from build123d import *

# Parameters (mm, degrees)
CROQUIS1_R              = 2
CROQUIS1_R_2            = 6
CROQUIS1_R_3            = 1
SALIENTE_EXTRUIR1_DEPTH = 6


with BuildPart() as part:
    # Croquis1 → Saliente-Extruir1 (new body)
    with BuildSketch(Plane.XY):
        with BuildLine():
            Line((-26.32, 5.852999231), (-2.53, 11.218248526))
            ThreePointArc((-2.53, 11.218248526), (0, 11.5), (2.53, 11.218248526))
            Line((2.53, 11.218248526), (26.32, 5.852999231))
            ThreePointArc((26.32, 5.852999231), (31, 0), (26.32, -5.852999231))
            Line((26.32, -5.852999231), (2.53, -11.218248526))
            ThreePointArc((2.53, -11.218248526), (0, -11.5), (-2.53, -11.218248526))
            Line((-2.53, -11.218248526), (-26.32, -5.852999231))
            ThreePointArc((-26.32, -5.852999231), (-31, 0), (-26.32, 5.852999231))
        make_face()
        with Locations((-25, 0)):
            Circle(CROQUIS1_R, mode=Mode.SUBTRACT)
        Circle(CROQUIS1_R_2, mode=Mode.SUBTRACT)
        with Locations((-16, 0)):
            Circle(CROQUIS1_R_3, mode=Mode.SUBTRACT)
        with Locations(Location((16, 0, 0), (0, 0, 180))):
            Circle(CROQUIS1_R_3, mode=Mode.SUBTRACT)
    extrude(amount=SALIENTE_EXTRUIR1_DEPTH)


solid = part.part
Part model, mm, in its own coordinate system. Give positions to 0.01 mm unless a question says otherwise; leave off trailing zeros. Loops run counter-clockwise (first coordinate to the right, second up) from the corner with the lowest first, then second, coordinate; pieces in that order, holes last. Notation, with made-up numbers: (51, -9) -> (77, -9) arc R26 ccw to (77, 28) -> close; hole circle Ø9 at (87, -7.5). An arc over 180 degrees is marked (long way). Write each question's results on one line, items separated by ' | '. Start each with the question number.
Q1. Pin check, flat tips, straight feed: P1, Ø6, axis at x = 23.5, y = 1.5, coming from the -Z side; P2, Ø3, axis at y = -3, z = 1, coming from the -X side; P3, Ø11, axis at x = 0, y = 0, coming from the -Z side. Stop position of each tip, or through.
Q2. Wall check: L1, parallel to Y at x = 0, z = 2.1; L2, parallel to Y at x = 5.5, z = 1.65; L3, parallel to X at y = -4, z = 2.05. Give the ranges that are in metal, low to high.
Q3. Band-saw the part on B-B on x = 0. List the corners of the cut face in (y, z), plus the area to 3 significant figures.
Q4. Band-saw the part on C-C on y = 0. List the corners of the cut face in (x, z).
Q5. Band-saw the part on D-D on y = -4. List the corners of the cut face in (x, z).
Q6. Pull direction Y, two halves, no side cores. Call faces 1 (the face through (14.258, 8.573, 2.958)), 2 (the face through (0, -11.5, 3)), 3 (the face through (-15, 0, 3)): +Y half, -Y half, draft (parallel to the pull), parting line (faces both ways), or undercut.
Q7. Band-saw the part on A-A on z = 0.55. List the corners of the cut face in (x, y), plus the area to 3 significant figures.
Results are:
1) P1: stops at z = 0 | P2: stops at x = -30.81 | P3: passes through
2) L1: y = -11.5 to -6, 6 to 11.5 | L2: y = -10.55 to -2.4, 2.4 to 10.55 | L3: x = -29.47 to -4.47, 4.47 to 29.47
3) outline: (-11.5, 0) -> (-6, 0) -> (-6, 6) -> (-11.5, 6) -> close; (6, 0) -> (11.5, 0) -> (11.5, 6) -> (6, 6) -> close | area: 66.0 mm²
4) outline: (-31, 0) -> (-27, 0) -> (-27, 6) -> (-31, 6) -> close; (-23, 0) -> (-17, 0) -> (-17, 6) -> (-23, 6) -> close; (-15, 0) -> (-6, 0) -> (-6, 6) -> (-15, 6) -> close; (6, 0) -> (15, 0) -> (15, 6) -> (6, 6) -> close; (17, 0) -> (31, 0) -> (31, 6) -> (17, 6) -> close
5) outline: (-29.47, 0) -> (-4.47, 0) -> (-4.47, 6) -> (-29.47, 6) -> close; (4.47, 0) -> (29.47, 0) -> (29.47, 6) -> (4.47, 6) -> close
6) face 1: +Y half | face 2: -Y half | face 3: undercut
7) outline: (-26.32, -5.85) -> (-2.53, -11.22) arc R11.5 ccw to (2.53, -11.22) -> (26.32, -5.85) arc R6 ccw to (26.32, 5.85) -> (2.53, 11.22) arc R11.5 ccw to (-2.53, 11.22) -> (-26.32, 5.85) arc R6 ccw to start; hole circle Ø4 at (-25, 0); hole circle Ø2 at (-16, 0); hole circle Ø12 at (0, 0); hole circle Ø2 at (16, 0) | area: 877 mm²
